from build123d import *

# Parameters (mm, degrees)
F1_DEPTH = 10
F0_W     = 30
F0_H     = 5
F2_DEPTH = 35
F4_DEPTH = 10.001


with BuildPart() as f1:
    # F0 (on Front) → F1 (new body)
    with BuildSketch(Plane.XZ):
        Polygon((32.5, 0), (-7.5, 20), (-32.5, 20), (-32.5, 15), (-22.5, 15), (-22.5, -10), (7.5, -10), (7.5, -15), (-22.5, -15), (-22.5, -20), (32.5, -20), align=None)
    extrude(amount=F1_DEPTH)

    # F0 (on Front) → F2 (join)
    with BuildSketch(Plane.XZ):
        Polygon((-22.5, 15), (-32.5, 15), (-32.5, -20), (-22.5, -20), (-22.5, -15), (-22.5, -10), align=None)
        with Locations((-7.5, -12.5)):
            Rectangle(F0_W, F0_H)
    extrude(amount=F2_DEPTH)

    # F3 (on face) → F4 (cut, through all)
    with BuildSketch(Plane.XY.offset(-10)):
        Polygon((7.5, -10), (-22.5, -35), (7.5, -35), align=None)
    extrude(amount=-F4_DEPTH, mode=Mode.SUBTRACT)


solid = f1.part
Can you work these out from the model? Positions are in its coordinate system, mm. A direction names the side the tool comes from. Coordinates: 2 decimals unless noted, no trailing zeros. Order: outer loops, then holes, each group sorted by start corner. A loop starts at its lowest first (then second) coordinate and runs counter-clockwise, first axis right, second up. Notation, with made-up numbers: M 82,72.5 L 104,72.5 A32 ccw 104,111.5 Z; hole C 14,35 d8. An arc over 180 degrees is marked long. Answer as CSV lines item,"result".
(1) I'm going to push flat-ended pins straight in: pin 1 (7.5 mm diameter, centred on x = -11.5, y = -27.5, fed in from -Z); pin 2 (4 mm diameter, centred on y = -20.5, z = 14.5, fed in from +X); pin 3 (3 mm diameter, centred on y = -8.5, z = 4, fed in from +X). Where does each tip first touch, or does it pass through?
Geometry check:
pin 1,"z = -15"
pin 2,"x = -22.5"
pin 3,"x = 27.5"
(2) Suppose I cut it at A-A on y = -27. Please give me the cut outline in (x, z), plus the area to 3 significant figures.
Geometry check:
outline,"M -32.5,-20 L -22.5,-20 L -22.5,-15 L -12.9,-15 L -12.9,-10 L -22.5,-10 L -22.5,15 L -32.5,15 Z"
area,"398 mm^2"
(3) Please list where these lines run through material, in increasing order: L1, parallel to Z at x = -17, y = -25; L2, parallel to Y at x = -11.5, z = 16.5; L3, parallel to X at y = -20, z = 9.
Geometry check:
L1,"-15 to -10"
L2,"-10 to 0"
L3,"-32.5 to -22.5"
(4) On a 3-axis mill with a long thin cutter (end or side, diameter ignored), from which of +Z, -Z, +X, -X, +Y, -Y can I reach the whole of each face in a straight line? I mean faces 1 (the flat face through (-11, -20, -10)), 2 (the flat face through (-27, -22, 15)), 3 (the flat face through (-11, -20, -15)), 4 (the flat face through (-20, -5, 20)). Say none if no direction works.
Geometry check:
face 1,"+Z, +X, -Y"
face 2,"+Z, +X, -X, -Y"
face 3,"-Z, +X, -Y"
face 4,"+Z, +X, -X, +Y, -Y"
(5) Suppose I cut it at D-D on z = -6. Please give me the cut outline in (x, y), plus the area to 3 significant figures.
Geometry check:
outline,"M -32.5,-35 L -22.5,-35 L -22.5,-10 L 32.5,-10 L 32.5,0 L -32.5,0 Z"
area,"900 mm^2"
(6) Suppose I cut it at B-B on x = -4.5. Please give me the cut outline in (y, z).
Geometry check:
outline,"M -20,-15 L -10,-15 L -10,-20 L 0,-20 L 0,18.5 L -10,18.5 L -10,-10 L -20,-10 Z"
(7) Suppose I cut it at C-C on z = -13. Please give me the cut outline in (x, y).
Geometry check:
outline,"M -32.5,-35 L -22.5,-35 L 7.5,-10 L 32.5,-10 L 32.5,0 L -32.5,0 Z"
(8) If we mould it in two halves opening along X, with no side actions, what happens to faces 5 (the flat face through (-32.5, -17, 0)), 6 (the flat face through (-22.5, -22, -18)), 7 (the flat face through (0, 0, -4))? For each: released by +X, released by -X, zero draft, split by the parting line, or undercut.
Geometry check:
face 5,"released by -X"
face 6,"released by +X"
face 7,"zero draft"
